Here's how the part is built. I have some questions about the finished solid (model axes, mm). A direction names the side the tool comes from. Give positions to 0.01 mm unless a question says otherwise; leave off trailing zeros. Order: outer loops, then holes, each group sorted by start corner. A loop starts at its lowest first (then second) coordinate and runs counter-clockwise, first axis right, second up.
from build123d import *

# Parameters (mm, degrees)
SKETCH1_R           = 3
BOSS_EXTRUDE1_DEPTH = 55.7
SKETCH2_W           = 0.8
SKETCH2_H           = 4.1
CUT_EXTRUDE1_DEPTH  = 4
SKETCH3_W           = 0.15
SKETCH3_H           = 0.75
CHAMFER1_SIZE       = 0.5


with BuildPart() as part:
    # Sketch1 → Boss-Extrude1 (new body)
    with BuildSketch(Plane(origin=(0, 0, 0), x_dir=(1, 0, 0), z_dir=(0, 1, 0))):
        Circle(SKETCH1_R)
    extrude(amount=BOSS_EXTRUDE1_DEPTH)

    # Sketch2 → Cut-Extrude1 (cut, symmetric)
    with BuildSketch(Plane.XY):
        with Locations((-2.6, 5.95)):
            Rectangle(SKETCH2_W, SKETCH2_H)
    cut_extrude1 = extrude(amount=CUT_EXTRUDE1_DEPTH, both=True, mode=Mode.SUBTRACT)

    # Mirror1: Cut-Extrude1 across plane
    add(cut_extrude1.mirror(Plane(origin=(0, 0, 0), x_dir=(0, 0, 1), z_dir=(1, 0, 0))), mode=Mode.SUBTRACT)

    # Sketch3 → Cut-Revolve1 (revolve, cut)
    with BuildSketch(Plane.XY):
        with Locations((2.925, 30.625)):
            Rectangle(SKETCH3_W, SKETCH3_H)
    revolve(axis=Axis((0, 55.7, 0), (0, -1, 0)), mode=Mode.SUBTRACT)

    # Chamfer1
    chamfer1_edges = [part.edges().sort_by_distance(p)[0] for p in [
        (-3, 0, 0),
        (-3, 55.7, 0),
    ]]
    chamfer(chamfer1_edges, length=CHAMFER1_SIZE)


solid = part.part
Q1. I need wall thicknesses on L1, parallel to Z at x = 0.1, y = 37; L2, parallel to X at y = 30, z = -0.95; L3, parallel to X at y = 50.5, z = -2.05. Which ranges of each line are inside material? Lowest first, please.
Filled sheet:
L1: z = -3 to 3
L2: x = -2.85 to 2.85
L3: x = -2.19 to 2.19
Q2. I'm going to push flat-ended pins straight in: P1, Ø3.5, axis at y = 6, z = 0, coming from the -X side; P2, Ø0.6, axis at x = -2.5, z = 0, coming from the -Y side; P3, Ø1.5, axis at y = 39.5, z = -1.5, coming from the +X side; P4, Ø1.2, axis at y = 7, z = 0, coming from the +X side. Where does each tip first touch, or does it pass through?
Filled sheet:
P1: stops at x = -2.2
P2: stops at y = 0
P3: stops at x = 2.9
P4: stops at x = 2.2
Q3. If we section it at A-A on z = 0: List the corners of the cut face in (x, y) for me, plus the area to 3 significant figures.
Filled sheet:
outline: (-3, 0.5) - (-2.5, 0) - (2.5, 0) - (3, 0.5) - (3, 3.9) - (2.2, 3.9) - (2.2, 8) - (3, 8) - (3, 30.25) - (2.85, 30.25) - (2.85, 31) - (3, 31) - (3, 55.2) - (2.5, 55.7) - (-2.5, 55.7) - (-3, 55.2) - (-3, 31) - (-2.85, 31) - (-2.85, 30.25) - (-3, 30.25) - (-3, 8) - (-2.2, 8) - (-2.2, 3.9) - (-3, 3.9) - close
area: 327 mm2
Q4. For faces 1 (the face through (-3, 43, 0)), 2 (the face through (2.2, 6, 0)), which set-ups out of +Z, -Z, +X, -X, +Y, -Y let a thin tool reach every point of the face, with its end or its side?
Filled sheet:
face 1: +Y, -Y
face 2: +Z, -Z, +X
Q5. Thinking about a two-plate mould opening in Y: for faces 3 (the face through (-2.262, 30.63, -1.734)), 4 (the face through (-2.2, 6, 0)), 5 (the face through (2.77, 15.17, 1.15)), 6 (the face through (0, 0, 0)), which applies, released by +Y, released by -Y, zero draft, split by the parting line, or undercut?
Filled sheet:
face 3: undercut
face 4: undercut
face 5: zero draft
face 6: released by -Y
Q6. If we section it at B-B on y = 52: List the corners of the cut face in (x, z) for me.
Filled sheet:
outline: circle Ø6 at (0, 0)
